The listing builds one solid part. Answer for the finished solid, in the listing's coordinates (mm). Give positions to 0.01 mm unless a question says otherwise; leave off trailing zeros. Write each loop counter-clockwise with the first axis right and the second up, starting at its lowest first coordinate (ties: lowest second). Pieces come first, ordered by that corner, then holes. Notation, with made-up numbers: (-14.75, 49.25) -> (-2.75, 49.25) arc R14 ccw to (-2.75, 67.25) -> close; hole circle Ø8 at (16, 76.25). An arc over 180 degrees is marked (long way). One line per question, with ' | ' between items.
from build123d import *

# Parameters (mm, degrees)
F0_W     = 120
F0_H     = 120
F0_R     = 2.5
F0_R_2   = 0.5
F1_DEPTH = 5


with BuildPart() as f1:
    # F0 (on Top) → F1 (new body)
    with BuildSketch(Plane.XY):
        Rectangle(F0_W, F0_H)
        with Locations((-52.5, -52.5)):
            Circle(F0_R, mode=Mode.SUBTRACT)
        with Locations((-19.103021, -26.293052)):
            Circle(F0_R_2, mode=Mode.SUBTRACT)
        with Locations((52.5, -52.5)):
            Circle(F0_R, mode=Mode.SUBTRACT)
        with Locations((19.103021, -26.293052)):
            Circle(F0_R_2, mode=Mode.SUBTRACT)
        with Locations((-30.909337, 10.043052)):
            Circle(F0_R_2, mode=Mode.SUBTRACT)
        with Locations((-52.5, 52.5)):
            Circle(F0_R, mode=Mode.SUBTRACT)
        with Locations((30.909337, 10.043052)):
            Circle(F0_R_2, mode=Mode.SUBTRACT)
        with Locations((0, 32.5)):
            Circle(F0_R_2, mode=Mode.SUBTRACT)
        with Locations((52.5, 52.5)):
            Circle(F0_R, mode=Mode.SUBTRACT)
    extrude(amount=F1_DEPTH)


solid = f1.part
Item 1: A flat-ended cylindrical pin translates along its axis: pin 1 (8 mm diameter, centred on x = 52.5, y = 52.5, fed in from -Z). Find the tip coordinate at first contact, or state that the pin passes through.
Answers below:
pin 1: z = 0
Item 2: Consider line 1 (Y direction, x = -52.5, z = 3); line 2 (X direction, y = 32.5, z = 1.55); line 3 (Y direction, x = -53, z = 3.6). Determine where each line is inside the solid, lowest interval first. Write a range as [from, to].
Answers below:
line 1: [-60, -55], [-50, 50], [55, 60] | line 2: [-60, -0.5], [0.5, 60] | line 3: [-60, -54.95], [-50.05, 50.05], [54.95, 60]
Item 3: Determine the mould class of faces 1 (the face through (-50.19, -53.46, 2.46)), 2 (the face through (-1, 1, 5)), 3 (the face through (-1, -60, 2)), 4 (the face through (-1, 60, 2)) for opening direction Y: pulls with the +Y half, pulls with the -Y half, needs draft (parallel to the pull), parting line crosses it, or undercut.
Answers below:
face 1: undercut | face 2: needs draft | face 3: pulls with the -Y half | face 4: pulls with the +Y half
Item 4: Find section A-A (x = 52.5). Write down the section's boundary in (y, z).
Answers below:
outline: (-60, 0) -> (-55, 0) -> (-55, 5) -> (-60, 5) -> close; (-50, 0) -> (50, 0) -> (50, 5) -> (-50, 5) -> close; (55, 0) -> (60, 0) -> (60, 5) -> (55, 5) -> close
